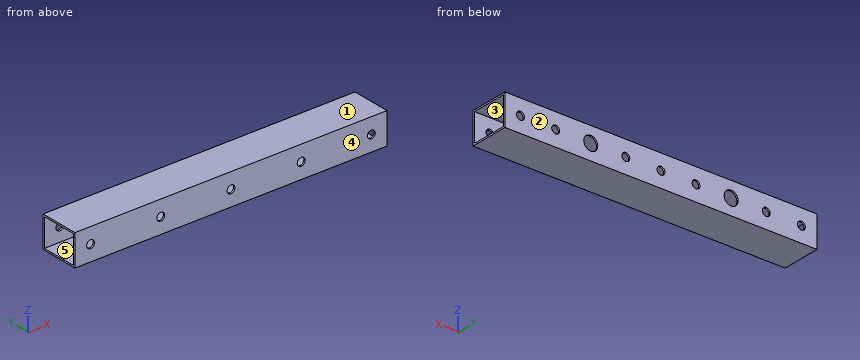
```python
from build123d import *

# Parameters (mm, degrees)
SKETCH_1_W          = 20
SKETCH_1_H          = 25
SKETCH_1_W_2        = 18
SKETCH_1_H_2        = 23
EXTRUDE_1_DEPTH     = 100
SKETCH_2_R          = 2.525
CUT_EXTRUDE_1_DEPTH = 5
SKETCH_4_R          = 2.5
CUT_EXTRUDE_3_DEPTH = 5
SKETCH_5_R          = 4.5
CUT_EXTRUDE_4_DEPTH = 2
SKETCH_6_R          = 2.525
CUT_EXTRUDE_5_DEPTH = 2
SKETCH_7_R          = 2.525
CUT_EXTRUDE_6_DEPTH = 10


with BuildPart() as part:
    # 草图1 → 凸台-拉伸1 (new, symmetric)
    with BuildSketch(Plane(origin=(0, 0, 0), x_dir=(0, 0, -1), z_dir=(1, 0, 0))):
        Rectangle(SKETCH_1_W, SKETCH_1_H)
        Rectangle(SKETCH_1_W_2, SKETCH_1_H_2, mode=Mode.SUBTRACT)
    extrude(amount=EXTRUDE_1_DEPTH, both=True)

    # 草图2 → 切除-拉伸1 (cut, symmetric)
    with BuildSketch(Plane(origin=(0, 12.5, 0), x_dir=(1, 0, 0), z_dir=(0, 1, 0))):
        with Locations(Location((0, 0, 0), (0, 0, 90))):
            Circle(SKETCH_2_R)
        with Locations(Location((-90, 0, 0), (0, 0, 90))):
            Circle(SKETCH_2_R)
        with Locations(Location((90, 0, 0), (0, 0, 90))):
            Circle(SKETCH_2_R)
    extrude(amount=CUT_EXTRUDE_1_DEPTH, both=True, mode=Mode.SUBTRACT)

    # 草图4 → 切除-拉伸3 (cut, symmetric)
    with BuildSketch(Plane(origin=(0, -11.5, 0), x_dir=(1, 0, 0), z_dir=(0, 1, 0))):
        with Locations(Location((-90, 0, 0), (0, 0, 270))):
            Circle(SKETCH_4_R)
        with Locations(Location((0, 0, 0), (0, 0, 270))):
            Circle(SKETCH_4_R)
        with Locations(Location((90, 0, 0), (0, 0, 270))):
            Circle(SKETCH_4_R)
    extrude(amount=CUT_EXTRUDE_3_DEPTH, both=True, mode=Mode.SUBTRACT)

    # 草图5 → 切除-拉伸4 (cut)
    with BuildSketch(Plane(origin=(0, 12.5, 0), x_dir=(1, 0, 0), z_dir=(0, 1, 0))):
        with Locations(Location((-45, 0, 0), (0, 0, 270))):
            Circle(SKETCH_5_R)
        with Locations(Location((45, 0, 0), (0, 0, 270))):
            Circle(SKETCH_5_R)
    extrude(amount=-CUT_EXTRUDE_4_DEPTH, mode=Mode.SUBTRACT)

    # 草图6 → 切除-拉伸5 (cut)
    with BuildSketch(Plane(origin=(0, -11.5, 0), x_dir=(1, 0, 0), z_dir=(0, 1, 0))):
        with Locations(Location((-45, 0, 0), (0, 0, 270))):
            Circle(SKETCH_6_R)
        with Locations(Location((45, 0, 0), (0, 0, 270))):
            Circle(SKETCH_6_R)
    extrude(amount=-CUT_EXTRUDE_5_DEPTH, mode=Mode.SUBTRACT)

    # 草图7 → 切除-拉伸6 (cut)
    with BuildSketch(Plane(origin=(0, 12.5, 0), x_dir=(1, 0, 0), z_dir=(0, 1, 0))):
        with Locations(Location((-67.5, 0, 0), (0, 0, 270))):
            Circle(SKETCH_7_R)
        with Locations(Location((-22.5, 0, 0), (0, 0, 270))):
            Circle(SKETCH_7_R)
        with Locations(Location((22.5, 0, 0), (0, 0, 270))):
            Circle(SKETCH_7_R)
        with Locations(Location((67.5, 0, 0), (0, 0, 270))):
            Circle(SKETCH_7_R)
    extrude(amount=-CUT_EXTRUDE_6_DEPTH, mode=Mode.SUBTRACT)


solid = part.part
```
Verification items for the finished model (mm, model axes). Face numbers are marked on the shaded views. A direction names the side the tool comes from. Give positions to 0.01 mm unless a question says otherwise; leave off trailing zeros. Loops run counter-clockwise (first coordinate to the right, second up) from the corner with the lowest first, then second, coordinate; pieces in that order, holes last.
1. Mould release check, pull along Z, two halves, no side actions. Record for the marked faces 1, 2 and 3: released by +Z, released by -Z, zero draft, split by the parting line, or undercut.
2. Section check B-B, the plane y = 1.5. Enter the section's corners in (x, z), then the cut area to 3 significant figures.
3. Set-up check for the marked faces 4 and 5: record each of +Z, -Z, +X, -X, +Y, -Y from which the full face is reachable in a straight line by a thin tool's end or side.
4. Go/stop test with flat-tipped pins: pin 1 Ø4 at (x, z) = (-90, 0) entering from -Y; pin 2 Ø5.5 at (x, z) = (-45, 0) entering from +Y. Record where each tip stops, or that it passes through.
5. Section check C-C, the plane x = -22.5. Enter the section's corners in (y, z) (3 decimals), then the cut area to 4 significant figures.
6. Section check D-D, the plane z = 0. Count the separate pieces of the cut face and the enclosed holes in it, then the cut area to 3 significant figures.
7. Thickness scan on line 1 (Y direction, x = -65.5, z = -7.5); line 2 (Z direction, x = 71.5, y = -9.75); line 3 (Y direction, x = -69.5, z = -1.25). Record the ranges inside material, lowest first.
8. Section check A-A, the plane x = 62. Enter the section's corners in (y, z), then the cut area to 3 significant figures.
Geometry says:
1. face 1: released by +Z
1. face 2: zero draft
1. face 3: undercut
2. outline: (-100, -10) - (100, -10) - (100, -9) - (-100, -9) - close; (-100, 9) - (100, 9) - (100, 10) - (-100, 10) - close
2. area: 400 mm2
3. face 4: +Z, -Z, +X, -X, -Y
3. face 5: +X, -X
4. pin 1: passes through
4. pin 2: stops at y = -11.5
5. outline: (-12.5, -10) - (12.5, -10) - (12.5, -2.525) - (11.5, -2.525) - (11.5, -9) - (-11.5, -9) - (-11.5, 9) - (11.5, 9) - (11.5, 2.525) - (12.5, 2.525) - (12.5, 10) - (-12.5, 10) - close
5. area: 80.95 mm2
6. separate pieces: 16
6. enclosed holes: 0
6. area: 322 mm2
7. line 1: y = -12.5 to -11.5, 11.5 to 12.5
7. line 2: z = -10 to -9, 9 to 10
7. line 3: y = -12.5 to -11.5
8. outline: (-12.5, -10) - (12.5, -10) - (12.5, 10) - (-12.5, 10) - close; hole (-11.5, -9) - (11.5, -9) - (11.5, 9) - (-11.5, 9) - close
8. area: 86.0 mm2
